```python
from build123d import *

# Parameters (mm, degrees)
F1_DEPTH = 24
F2_R     = 13
F3_R     = 5
F5_DEPTH = 11
F6_R     = 2.5
F7_DEPTH = 41.001
F8_R     = 5
F9_DEPTH = 11.001
F10_R    = 2


with BuildPart() as f1:
    # F0 (on Right) → F1 (new body, symmetric)
    with BuildSketch(Plane.YZ):
        with BuildLine():
            Line((0, 41), (0, 0))
            Line((0, 0), (34.45, 0))
            ThreePointArc((34.45, 0), (53.5, 19.05), (72.55, 0))
            Line((72.55, 0), (107, 0))
            Line((107, 0), (107, 11))
            Line((107, 11), (81.410571, 11))
            ThreePointArc((81.410571, 11), (53.5, 30), (25.589429, 11))
            Line((25.589429, 11), (11, 11))
            Line((11, 11), (11, 41))
            Line((11, 41), (0, 41))
        make_face()
    extrude(amount=F1_DEPTH, both=True)

    # F2
    f2_edges = [f1.edges().sort_by_distance(p)[0] for p in [
        (24, 107, 5.5),
        (-24, 107, 5.5),
    ]]
    fillet(f2_edges, radius=F2_R)

    # F3
    f3_edges = [f1.edges().sort_by_distance(p)[0] for p in [
        (-24, 5.5, 41),
        (24, 5.5, 41),
    ]]
    fillet(f3_edges, radius=F3_R)

    # F4 (on face) → F5 (cut, through all)
    with BuildSketch(Plane.XZ):
        with BuildLine():
            Line((-6.5, 41), (-6.5, 25))
            ThreePointArc((-6.5, 25), (0, 18.5), (6.5, 25))
            Line((6.5, 25), (6.5, 41))
            Line((6.5, 41), (-6.5, 41))
        make_face()
    extrude(amount=-F5_DEPTH, mode=Mode.SUBTRACT)

    # F6 (on Top) → F7 (cut, through all)
    with BuildSketch(Plane.XY):
        with Locations((0, 51)):
            Circle(F6_R)
    extrude(amount=F7_DEPTH, mode=Mode.SUBTRACT)

    # F8 (on face) → F9 (cut, through all)
    with BuildSketch(Plane.XY.offset(11)):
        with Locations((-11, 96.5)):
            Circle(F8_R)
        with Locations((11, 96.5)):
            Circle(F8_R)
    extrude(amount=-F9_DEPTH, mode=Mode.SUBTRACT)

    # F10
    f10_edges = [f1.edges().sort_by_distance(p)[0] for p in [
        (0, 25.589429, 11),
        (0, 81.410571, 11),
    ]]
    fillet(f10_edges, radius=F10_R)


solid = f1.part
```
Design review of the part built by this model. Coordinates are the model's own, in mm. A direction names the side the tool comes from. Coordinates: 2 decimals unless noted, no trailing zeros. Write each loop counter-clockwise with the first axis right and the second up, starting at its lowest first coordinate (ties: lowest second). Pieces come first, ordered by that corner, then holes.
1) Machinability: for faces 4 (the flat face through (6, 11, 19)), 5 (the flat face through (0, 95, 11)), 6 (the flat face through (6.5, 5, 33)), 7 (the cylindrical face through (20.091, 103.293, 5.577)), which of the approach directions +Z, -Z, +X, -X, +Y, -Y give a long, thin tool a straight path to every point of the face, cutting with its end or side? Answer none if there is none.
2) Add section B-B (z = 9). Write out the cut boundary in (x, y), plus the area to 3 significant figures.
3) Insertion check: pin 1 (1 mm diameter, centred on x = -17.5, y = 62, fed in from +Z); pin 2 (4 mm diameter, centred on x = 16, z = 11, fed in from +Y); pin 3 (13 mm diameter, centred on x = 11, y = 96.5, fed in from +Z); pin 4 (8 mm diameter, centred on x = -11, y = 96.5, fed in from -Z). Each pin has a flat end and moves straight along its axis. Give the tip position at first contact, or say it passes through.
4) Mouldability with a two-part tool opening along X and no side actions: class faces 1 (the cylindrical face through (-0.1, 5.4, 18.5)), 2 (the flat face through (24, 36, 14)), 3 (the flat face through (0, 18, 11)) as +X half, -X half, draft (parallel to the pull), parting line (faces both ways), or undercut.
5) To check wall thickness, follow L1, parallel to X at y = 96, z = 8; L2, parallel to Y at x = -15.5, z = 11.5; L3, parallel to Y at x = -11, z = 7.5. State the ranges of each line that lie inside material, in increasing order.
6) Add section C-C (x = -1.5). Write out the cut boundary in (y, z), plus the area to 3 significant figures.
7) Add section A-A (y = 51). Write out the cut boundary in (x, z).
8) Add section D-D (z = 13.5). Write out the cut boundary in (x, y).
Check result:
1. face 4: +Z, +X, -X
1. face 5: +Z, +X, -X, +Y
1. face 6: +Z, -Y
1. face 7: +Z, -Z, +X, +Y
2. outline: (-24, 0) - (24, 0) - (24, 36.71) - (-24, 36.71) - close; (-24, 70.29) - (24, 70.29) - (24, 94) arc R13 ccw to (11, 107) - (-11, 107) arc R13 ccw to (-24, 94) - close; hole circle Ø10 at (-11, 96.5); hole circle Ø10 at (11, 96.5)
2. area: 3,290 mm2
3. pin 1: stops at z = 28.91
3. pin 2: stops at y = 106.65
3. pin 3: stops at z = 11
3. pin 4: passes through
4. face 1: undercut
4. face 2: +X half
4. face 3: draft
5. L1: x = -23.85 to -15.97, -6.03 to 6.03, 15.97 to 23.85
5. L2: y = 0 to 11, 25.58 to 38.31, 68.69 to 81.42
5. L3: y = 0 to 35.99, 71.01 to 91.5, 101.5 to 107
6. outline: (0, 0) - (34.45, 0) arc R19.05 cw to (49, 18.51) - (49, 29.66) arc R30 ccw to (26.09, 12.19) arc R2 cw to (24.26, 11) - (11, 11) - (11, 18.68) - (0, 18.68) - close; (53, 19.04) arc R19.05 cw to (72.55, 0) - (107, 0) - (107, 11) - (82.74, 11) arc R2 cw to (80.91, 12.19) arc R30 ccw to (53, 30) - close
6. area: 1,420 mm2
7. outline: (-24, 18.89) - (-2.5, 18.89) - (-2.5, 29.9) - (-24, 29.9) - close; (2.5, 18.89) - (24, 18.89) - (24, 29.9) - (2.5, 29.9) - close
8. outline: (-24, 0) - (24, 0) - (24, 11) - (-24, 11) - close; (-24, 26.71) - (24, 26.71) - (24, 40.06) - (-24, 40.06) - close; (-24, 66.94) - (24, 66.94) - (24, 80.29) - (-24, 80.29) - close
